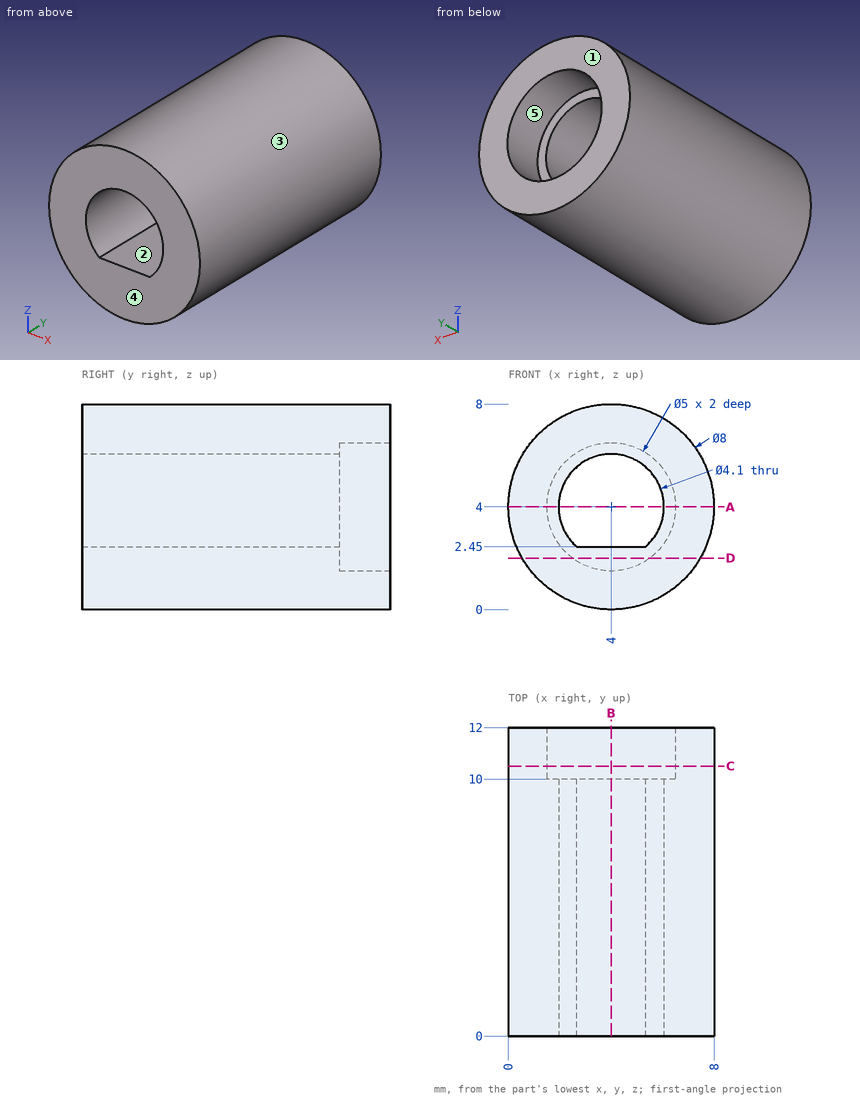
Geometry check sheet. Reference: drawing and pictorial views, mm from the part's lowest x, y, z. A direction names the side the tool comes from. Round coordinates to 2 decimals unless told otherwise and drop trailing zeros. Write each loop counter-clockwise with the first axis right and the second up, starting at its lowest first coordinate (ties: lowest second). Pieces come first, ordered by that corner, then holes. Notation, with made-up numbers: (-29, 46) -> (-13, 46) arc R5 ccw to (-13, 55) -> close; hole circle Ø9 at (-27.5, 50.25). An arc over 180 degrees is marked (long way). Answer as CSV lines item,"result". Start each with the question number.
1) Material ranges on line 1 (X direction, y = 11.35, z = 4); line 2 (X direction, y = 4, z = 4); line 3 (Y direction, x = 2.25, z = 5.5), recorded low to high. Write a range as from..to.
2) Section check D-D on z = 2. Enter the section's corners in (x, y).
3) Go/stop test with flat-tipped pins: P1, Ø3, axis at x = 1, y = 9.5, coming from the -Z side; P2, Ø3.5, axis at x = 4, z = 4, coming from the +Y side. Record where each tip stops, or that it passes through.
4) Tool access check on the marked faces 1 and 2. Record the directions out of +Z, -Z, +X, -X, +Y, -Y that give a thin tool (end or side, any length) a straight path to the whole face; none if there is none.
5) Section check C-C on y = 10.5. Enter the section's corners in (x, z), and give its area (3 significant figures).
6) Release check for a two-part mould opening along X. For the marked faces 3, 4 and 5 record: pulls with the +X half, pulls with the -X half, needs draft (parallel to the pull), parting line crosses it, or undercut.
7) Section check A-A on z = 4. Enter the section's corners in (x, y).
8) Section check B-B on x = 4. Enter the section's corners in (y, z), and give its area (3 significant figures).
Found:
1,line 1,"x = 0..1.5, 6.5..8"
1,line 2,"x = 0..1.95, 6.05..8"
1,line 3,"y = 0..10"
2,outline,"(0.54, 0) -> (7.46, 0) -> (7.46, 12) -> (5.5, 12) -> (5.5, 10) -> (2.5, 10) -> (2.5, 12) -> (0.54, 12) -> close"
3,P1,"stops at z = 0.29"
3,P2,"stops at y = 10"
4,face 1,"+Z, -Z, +X, -X, +Y"
4,face 2,"+Y, -Y"
5,outline,"circle Ø8 at (4, 4); hole circle Ø5 at (4, 4)"
5,area,"30.6 mm^2"
6,face 3,"parting line crosses it"
6,face 4,"needs draft"
6,face 5,"undercut"
7,outline,"(0, 0) -> (1.95, 0) -> (1.95, 10) -> (1.5, 10) -> (1.5, 12) -> (0, 12) -> close; (6.05, 0) -> (8, 0) -> (8, 12) -> (6.5, 12) -> (6.5, 10) -> (6.05, 10) -> close"
8,outline,"(0, 0) -> (12, 0) -> (12, 1.5) -> (10, 1.5) -> (10, 2.45) -> (0, 2.45) -> close; (0, 6.05) -> (10, 6.05) -> (10, 6.5) -> (12, 6.5) -> (12, 8) -> (0, 8) -> close"
8,area,"50.0 mm^2"
